Geometry: final body of the model. Coordinates: model frame, mm. Face numbers are marked on the shaded views. A direction names the side the tool comes from. Give positions to 0.01 mm unless a question says otherwise; leave off trailing zeros. Write each loop counter-clockwise with the first axis right and the second up, starting at its lowest first coordinate (ties: lowest second). Pieces come first, ordered by that corner, then holes. Notation, with made-up numbers: (80.5, 33) -> (136.5, 33) arc R15 ccw to (136.5, 62) -> close; hole circle Ø8 at (-27.75, 60.25). An arc over 180 degrees is marked (long way). Answer in a Markdown table with one row per item. Add a question column.
Item 1: Section query B-B on x = 24. Output: boundary loops of the cut face in (y, z).
Item 2: First-contact query: P1, Ø3.5, axis at x = 1.5, z = -21, coming from the +Y side; P2, Ø4, axis at x = -38, y = 8.5, coming from the +Z side; P3, Ø2, axis at x = 12.5, z = -23.5, coming from the +Y side. Flat tips, straight axial feed; report the tip coordinate or a pass-through.
Item 3: Section query A-A on z = -23. Output: boundary loops of the cut face in (x, y).
Item 4: Access query for the marked faces 5 and 6. Directions: +Z, -Z, +X, -X, +Y, -Y. A direction counts if a zero-diameter tool reaches every point of the face in a straight line with its end or side. Return the directions, or none.
Item 5: Section query D-D on z = 16. Output: boundary loops of the cut face in (x, y), plus the area to 3 significant figures.
Item 6: Material intervals for probe 1 along X at (y, z) = (8.25, -28); probe 2 along Z at (x, y) = (23.5, 7.25); probe 3 along X at (y, z) = (9.5, 30.5), sorted ascending. Write a range as from..to.
Item 7: Section query C-C on y = 15.5. State how many separate pieces and enclosed holes the cut face has, plus the area to 3 significant figures.
Item 8: Draft query along Z for the marked faces 1, 2, 3 and 4. Return one class per face: +Z half, -Z half, draft (parallel to the pull), parting line (faces both ways), or undercut.
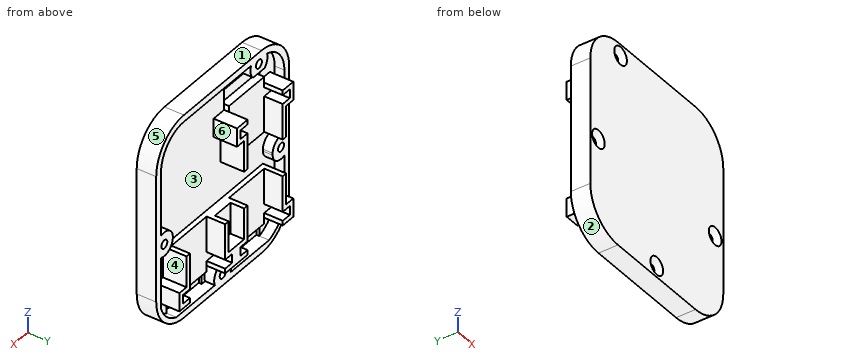
```python
from build123d import *

# Parameters (mm, degrees)
BASE_DEPTH                                        = 10
HOLE_FOR_ACTUATOR_COVERS_DEPTH                    = 5
SIDE_CLAMPS_DEPTH                                 = 7
SKETCH14_W                                        = 25.4
SKETCH14_H                                        = 7.5
PULLEY_CLEARANCES_DEPTH                           = 6.5
CSK_FOR_8_FLAT_HEAD_SOCKET_CAP_SCREW1_D           = 4.3053
CSK_FOR_8_FLAT_HEAD_SOCKET_CAP_SCREW1_CSINK_D     = 9.1186
CSK_FOR_8_FLAT_HEAD_SOCKET_CAP_SCREW1_CSINK_ANGLE = 82
ACTUATOR_GROOVE_DEPTH                             = 2.5
MATERIAL_CUTAWAY_DEPTH                            = 5


with BuildPart() as part:
    # Sketch1 → base (new body)
    with BuildSketch(Plane(origin=(0, 0, 0), x_dir=(1, 0, 0), z_dir=(0, 1, 0))):
        with BuildLine():
            Line((-28, 52.5), (28, 52.5))
            ThreePointArc((28, 52.5), (42.142135624, 46.642135624), (48, 32.5))
            Line((48, 32.5), (48, -32.5))
            ThreePointArc((48, -32.5), (42.142135624, -46.642135624), (28, -52.5))
            Line((28, -52.5), (-28, -52.5))
            ThreePointArc((-28, -52.5), (-42.142135624, -46.642135624), (-48, -32.5))
            Line((-48, -32.5), (-48, 32.5))
            ThreePointArc((-48, 32.5), (-42.142135624, 46.642135624), (-28, 52.5))
        make_face()
    extrude(amount=BASE_DEPTH)

    # Sketch10 → hole for actuator covers (cut)
    with BuildSketch(Plane(origin=(0, 10, 0), x_dir=(1, 0, 0), z_dir=(0, 1, 0))):
        Polygon((-5.6, 5.5), (-5.6, 13), (-8.6, 13), (-33, 13), (-36, 13), (-36, 5.5), align=None)
        Polygon((33, 13), (36, 13), (36, 5.5), (5.6, 5.5), (5.6, 13), (8.6, 13), align=None)
        Polygon((-5.6, -6), (-8.6, -6), (-33, -6), (-36, -6), (-36, 1.5), (-5.6, 1.5), align=None)
    extrude(amount=-HOLE_FOR_ACTUATOR_COVERS_DEPTH, mode=Mode.SUBTRACT)

    # Sketch13 → side clamps (add)
    with BuildSketch(Plane(origin=(0, 10, 0), x_dir=(1, 0, 0), z_dir=(0, 1, 0))):
        Polygon((-8.1, -24.45), (-3, -24.45), (-3, -29.05), (-8.1, -29.05), (-8.1, -31.5), (-0.5, -31.5), (-0.5, -22), (-5.6, -22), (-5.6, -6), (-8.1, -6), align=None)
        Polygon((-41.1, 29), (-41.1, 38.5), (-33.5, 38.5), (-33.5, 36.05), (-38.6, 36.05), (-38.6, 31.45), (-33.5, 31.45), (-33.5, 13), (-36, 13), (-36, 29), align=None)
        Polygon((-8.1, 13), (-8.1, 31.45), (-3, 31.45), (-3, 36.05), (-8.1, 36.05), (-8.1, 38.5), (8.1, 38.5), (8.1, 36.05), (3, 36.05), (3, 31.45), (8.1, 31.45), (8.1, 13), (5.6, 13), (5.6, 29), (-5.6, 29), (-5.6, 13), align=None)
        Polygon((33.5, 13), (33.5, 31.45), (38.6, 31.45), (38.6, 36.05), (33.5, 36.05), (33.5, 38.5), (41.1, 38.5), (41.1, 29), (36, 29), (36, 13), align=None)
        Polygon((-38.6, -24.45), (-38.6, -29.05), (-33.5, -29.05), (-33.5, -31.5), (-41.1, -31.5), (-41.1, -22), (-36, -22), (-36, -6), (-33.5, -6), (-33.5, -24.45), align=None)
    extrude(amount=SIDE_CLAMPS_DEPTH)

    # Sketch14 → pulley clearances (cut)
    with BuildSketch(Plane(origin=(0, 10, 0), x_dir=(1, 0, 0), z_dir=(0, 1, 0))):
        with Locations((-20.8, -38.3)):
            Rectangle(SKETCH14_W, SKETCH14_H)
        with Locations((-20.8, 45.3)):
            Rectangle(SKETCH14_W, SKETCH14_H)
        with Locations((20.8, 45.3)):
            Rectangle(SKETCH14_W, SKETCH14_H)
    extrude(amount=-PULLEY_CLEARANCES_DEPTH, mode=Mode.SUBTRACT)

    # CSK for #8 Flat Head Socket Cap Screw1 (through all)
    with Locations(Plane(origin=(0, 0, 0), x_dir=(-1, 0, 0), z_dir=(0, -1, 0))):
        with Locations((26.142135624, -46.642135624), (42.142135624, 6), (0, 46.642135624), (-42.142135624, 6)):
            CounterSinkHole(CSK_FOR_8_FLAT_HEAD_SOCKET_CAP_SCREW1_D / 2, CSK_FOR_8_FLAT_HEAD_SOCKET_CAP_SCREW1_CSINK_D / 2, counter_sink_angle=CSK_FOR_8_FLAT_HEAD_SOCKET_CAP_SCREW1_CSINK_ANGLE)

    # Sketch18 → actuator groove (cut)
    with BuildSketch(Plane(origin=(0, 10, 0), x_dir=(1, 0, 0), z_dir=(0, 1, 0))):
        Polygon((-33.5, 31.45), (-33.5, 13), (-8.1, 13), (-8.1, 31.45), (-3, 31.45), (-3, 36.05), (-8.1, 36.05), (-8.1, 41.55), (-33.5, 41.55), (-33.5, 36.05), (-38.6, 36.05), (-38.6, 31.45), align=None)
        Polygon((38.6, 31.45), (38.6, 36.05), (33.5, 36.05), (33.5, 41.55), (8.1, 41.55), (8.1, 36.05), (3, 36.05), (3, 31.45), (8.1, 31.45), (8.1, 13), (33.5, 13), (33.5, 31.45), align=None)
        Polygon((-33.5, -6), (-33.5, -24.45), (-38.6, -24.45), (-38.6, -29.05), (-33.5, -29.05), (-33.5, -34.55), (-8.1, -34.55), (-8.1, -29.05), (-3, -29.05), (-3, -24.45), (-8.1, -24.45), (-8.1, -6), align=None)
    extrude(amount=-ACTUATOR_GROOVE_DEPTH, mode=Mode.SUBTRACT)

    # Sketch20 → material cutaway (cut)
    with BuildSketch(Plane(origin=(0, 10, 0), x_dir=(1, 0, 0), z_dir=(0, 1, 0))):
        with BuildLine():
            Line((-36, -6), (-5.6, -6))
            Line((-5.6, -6), (-5.6, -22))
            Line((-5.6, -22), (-0.5, -22))
            Line((-0.5, -22), (-0.5, -31.5))
            Line((-0.5, -31.5), (-8.1, -31.5))
            Line((-8.1, -31.5), (-8.1, -42.05))
            Line((-8.1, -42.05), (-22.032619784, -42.05))
            ThreePointArc((-22.032619784, -42.05), (-20.127795479, -45.29917522), (-20.469568377, -49.05))
            Line((-20.469568377, -49.05), (28, -49.05))
            ThreePointArc((28, -49.05), (39.702617229, -44.202617229), (44.55, -32.5))
            Line((44.55, -32.5), (44.55, 0.327432754))
            ThreePointArc((44.55, 0.327432754), (38.952298885, 0.727356298), (36, 5.5))
            ThreePointArc((36, 5.5), (38.535011833, 10.996447536), (44.55, 11.672567246))
            Line((44.55, 11.672567246), (44.55, 37.948525732))
            ThreePointArc((44.55, 37.948525732), (40.344819956, 44.812963205), (33.5, 49.05))
            Line((33.5, 49.05), (8.1, 49.05))
            Line((8.1, 49.05), (5.672567246, 49.05))
            ThreePointArc((5.672567246, 49.05), (0, 40.479682377), (-5.672567246, 49.05))
            Line((-5.672567246, 49.05), (-8.1, 49.05))
            Line((-8.1, 49.05), (-33.5, 49.05))
            ThreePointArc((-33.5, 49.05), (-40.344819956, 44.812963205), (-44.55, 37.948525732))
            Line((-44.55, 37.948525732), (-44.55, 11.672567246))
            ThreePointArc((-44.55, 11.672567246), (-35.979682377, 6), (-44.55, 0.327432754))
            Line((-44.55, 0.327432754), (-44.55, -32.5))
            ThreePointArc((-44.55, -32.5), (-41.039944494, -42.691287828), (-31.998658901, -48.559677051))
            ThreePointArc((-31.998658901, -48.559677051), (-32.093980526, -45.044834063), (-30.251651463, -42.05))
            Line((-30.251651463, -42.05), (-33.5, -42.05))
            Line((-33.5, -42.05), (-33.5, -31.5))
            Line((-33.5, -31.5), (-41.1, -31.5))
            Line((-41.1, -31.5), (-41.1, -22))
            Line((-41.1, -22), (-36, -22))
            Line((-36, -22), (-36, -6))
        make_face()
        Polygon((-8.1, 38.5), (-8.1, 41.55), (-33.5, 41.55), (-33.5, 38.5), (-41.1, 38.5), (-41.1, 29), (-36, 29), (-36, 13), (36, 13), (36, 29), (41.1, 29), (41.1, 38.5), (33.5, 38.5), (33.5, 41.55), (8.1, 41.55), (8.1, 38.5), align=None, mode=Mode.SUBTRACT)
    extrude(amount=-MATERIAL_CUTAWAY_DEPTH, mode=Mode.SUBTRACT)


solid = part.part
```
Findings below:
| question | item | result |
|---|---|---|
| 1 | outline | (0, -52.5) -> (10, -52.5) -> (10, -49.05) -> (3.5, -49.05) -> (3.5, -41.55) -> (7.5, -41.55) -> (7.5, -13) -> (5, -13) -> (5, 49.05) -> (10, 49.05) -> (10, 52.5) -> (0, 52.5) -> close |
| 2 | P1 | stops at y = 10 |
| 2 | P2 | stops at z = 50.83 |
| 2 | P3 | stops at y = 7.5 |
| 3 | outline | (-48, 0) -> (48, 0) -> (48, 10) -> (44.55, 10) -> (44.55, 5) -> (36, 5) -> (36, 17) -> (33.5, 17) -> (33.5, 7.5) -> (8.1, 7.5) -> (8.1, 17) -> (5.6, 17) -> (5.6, 10) -> (-5.6, 10) -> (-5.6, 17) -> (-8.1, 17) -> (-8.1, 7.5) -> (-33.5, 7.5) -> (-33.5, 17) -> (-36, 17) -> (-36, 5) -> (-44.55, 5) -> (-44.55, 10) -> (-48, 10) -> close |
| 4 | face 5 | +Z, +X, +Y, -Y |
| 4 | face 6 | +Y |
| 5 | outline | (-48, 0) -> (48, 0) -> (48, 10) -> (44.55, 10) -> (44.55, 5) -> (-5.6, 5) -> (-5.6, 17) -> (-8.1, 17) -> (-8.1, 7.5) -> (-33.5, 7.5) -> (-33.5, 17) -> (-36, 17) -> (-36, 5) -> (-44.55, 5) -> (-44.55, 10) -> (-48, 10) -> close |
| 5 | area | 638 mm^2 |
| 6 | probe 1 | x = -48..-44.55, -36..-33.5, -8.1..8.1, 33.5..36, 44.55..48 |
| 6 | probe 2 | z = -52.5..-49.05, -41.55..-13, 49.05..52.5 |
| 6 | probe 3 | x = -48..-44.55, -41.1..-33.5, -8.1..-0.5, 44.55..48 |
| 7 | separate pieces | 5 |
| 7 | enclosed holes | 0 |
| 7 | area | 542 mm^2 |
| 8 | face 1 | +Z half |
| 8 | face 2 | -Z half |
| 8 | face 3 | undercut |
| 8 | face 4 | undercut |
